Could you check a few things on this model? Use its own coordinates, in mm. Face numbers are marked on the shaded views. Round coordinates to 2 decimals unless told otherwise and drop trailing zeros. Write each loop counter-clockwise with the first axis right and the second up, starting at its lowest first coordinate (ties: lowest second). Pieces come first, ordered by that corner, then holes. Notation, with made-up numbers: (-22, 1) -> (6, 1) arc R11 ccw to (6, 17) -> close; hole circle Ø2 at (79, 5.5). An arc over 180 degrees is marked (long way). Answer in a Markdown table with one row per item. Add a question column.
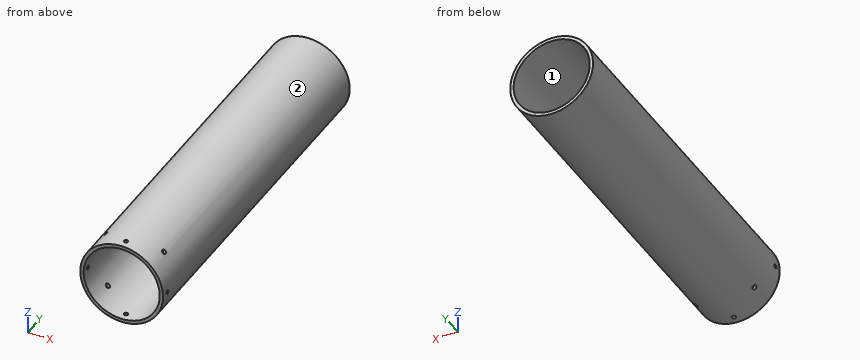
```python
from build123d import *

# Parameters (mm, degrees)
SKETCH_1_R               = 25
SKETCH_1_R_2             = 23
EXTRUDE_1_DEPTH          = 214
SKETCH_5_R               = 1.2
CUT_EXTRUDE_5_DEPTH      = 217.90089903
PATTERN_CIRCULAR_1_COUNT = 4
SKETCH_6_R               = 1.4
CUT_EXTRUDE_6_DEPTH      = 217.900899153
PATTERN_CIRCULAR_2_COUNT = 4


with BuildPart() as part:
    # Эскиз1 → Бобышка-Вытянуть1 (new body)
    with BuildSketch(Plane(origin=(0, 0, 0), x_dir=(1, 0, 0), z_dir=(0, 1, 0))):
        with Locations(Location((0, 0, 0), (0, 0, 270))):
            Circle(SKETCH_1_R)
        with Locations(Location((0, 0, 0), (0, 0, 270))):
            Circle(SKETCH_1_R_2, mode=Mode.SUBTRACT)
    extrude(amount=EXTRUDE_1_DEPTH)

    # Эскиз5 → Вырез-Вытянуть5 (cut, through all)
    with BuildSketch(Plane.XY):
        with Locations(Location((0, 5, 0), (0, 0, 90))):
            Circle(SKETCH_5_R)
    cut_extrude_5 = extrude(amount=-CUT_EXTRUDE_5_DEPTH, mode=Mode.SUBTRACT)

    # Круговой массив1: Вырез-Вытянуть5 ×4 about axis
    pattern_circular_1_axis = Axis((0, 214, 0), (0, -1, 0))
    for i in range(1, PATTERN_CIRCULAR_1_COUNT):
        add(cut_extrude_5.rotate(pattern_circular_1_axis, i * 360 / PATTERN_CIRCULAR_1_COUNT), mode=Mode.SUBTRACT)

    # Эскиз6 → Вырез-Вытянуть6 (cut, through all)
    with BuildSketch(Plane(origin=(0, 0, 0), x_dir=(0, -1, 0), z_dir=(-0.7071067811865488, 0, 0.7071067811865464))):
        with Locations(Location((-15, 0, 0), (0, 0, 90))):
            Circle(SKETCH_6_R)
    cut_extrude_6 = extrude(amount=-CUT_EXTRUDE_6_DEPTH, mode=Mode.SUBTRACT)

    # Круговой массив2: Вырез-Вытянуть6 ×4 about axis
    pattern_circular_2_axis = Axis((0, 214, 0), (0, -1, 0))
    for i in range(1, PATTERN_CIRCULAR_2_COUNT):
        add(cut_extrude_6.rotate(pattern_circular_2_axis, i * 360 / PATTERN_CIRCULAR_2_COUNT), mode=Mode.SUBTRACT)


solid = part.part
```
(1) I need wall thicknesses on L1, parallel to Y at x = 0, z = 24; L2, parallel to Z at x = -11, y = 135.5; L3, parallel to Z at x = 15, y = 202. Which ranges of each line are inside material? Lowest first, please.
(2) Suppose I cut it at B-B, the plane x = -8. Please give me the cut outline in (y, z).
(3) Suppose I cut it at A-A, the plane z = -20.5. Please give me the cut outline in (x, y).
(4) Suppose I cut it at C-C, the plane y = 21.5. Please give me the cut outline in (x, z), then the cut area to 3 significant figures.
(5) For P1, Ø1.5, axis at y = 167, z = -4, coming from the +X side; P2, Ø5, axis at x = 4, y = 152.5, coming from the -Z side; P3, Ø1.5, axis at x = 9, y = 36, coming from the +Z side, each with a flat end and sliding along its axis, tell me the tip position at first contact or that it passes through.
(6) If we mould it in two halves opening along X, with no side actions, what happens to the marked faces 1 and 2? For each: pulls with the +X half, pulls with the -X half, needs draft (parallel to the pull), parting line crosses it, or undercut.
Response:
| question | item | result |
|---|---|---|
| 1 | L1 | 0 to 3.8, 6.2 to 214 |
| 1 | L2 | -22.45 to -20.2, 20.2 to 22.45 |
| 1 | L3 | -20 to -17.44, 17.44 to 20 |
| 2 | outline | (0, -23.69) -> (214, -23.69) -> (214, -21.56) -> (0, -21.56) -> close; (0, 21.56) -> (214, 21.56) -> (214, 23.69) -> (0, 23.69) -> close |
| 3 | outline | (-14.31, 0) -> (-10.43, 0) -> (-10.43, 214) -> (-14.31, 214) -> close; (10.43, 0) -> (14.31, 0) -> (14.31, 214) -> (10.43, 214) -> close |
| 4 | outline | circle Ø50 at (0, 0); hole circle Ø46 at (0, 0) |
| 4 | area | 302 mm² |
| 5 | P1 | x = 24.79 |
| 5 | P2 | z = -24.95 |
| 5 | P3 | z = 23.6 |
| 6 | face 1 | undercut |
| 6 | face 2 | parting line crosses it |
